Input: dimensioned drawing with shaded views. Units: mm. Origin: part minimum x, y, z. A direction names the side the tool comes from. Round coordinates to 2 decimals unless told otherwise and drop trailing zeros. Order: outer loops, then holes, each group sorted by start corner. A loop starts at its lowest first (then second) coordinate and runs counter-clockwise, first axis right, second up. Notation, with made-up numbers: M 11,-22.75 L 23,-22.75 A19 ccw 23,-12.75 Z; hole C 11,59 d1. An arc over 180 degrees is marked long. Put each result on its own line as item: value. Start each with the question number.
1) Section D-D, the plane y = 52.5. Return loops of the section in (x, z), then the cut area to 3 significant figures.
2) Access query for the marked faces 5 and 6. Directions: +Z, -Z, +X, -X, +Y, -Y. A direction counts if a zero-diameter tool reaches every point of the face in a straight line with its end or side. Return the directions, or none.
3) Section A-A, the plane z = 27.5. Return loops of the section in (x, y), then the cut area to 3 significant figures.
4) Section B-B, the plane y = 71. Return loops of the section in (x, z).
5) Draft query along X for the marked faces 1, 2, 3 and 4. Return one class per face: pulls with the +X half, pulls with the -X half, needs draft (parallel to the pull), parting line crosses it, or undercut.
6) Material intervals for probe 1 along Z at (x, y) = (26.15, 2.9); probe 2 along X at (y, z) = (2.05, 12.5); probe 3 along X at (y, z) = (7, 8), sorted ascending. Write a range as [from, to].
7) First-contact query: P1, Ø4, axis at x = 56.15, z = 42.5, coming from the +Y side. Flat tip, straight axial feed; report the tip coordinate or a pass-through.
8) Section C-C, the plane x = 56.15. Return loops of the section in (y, z).
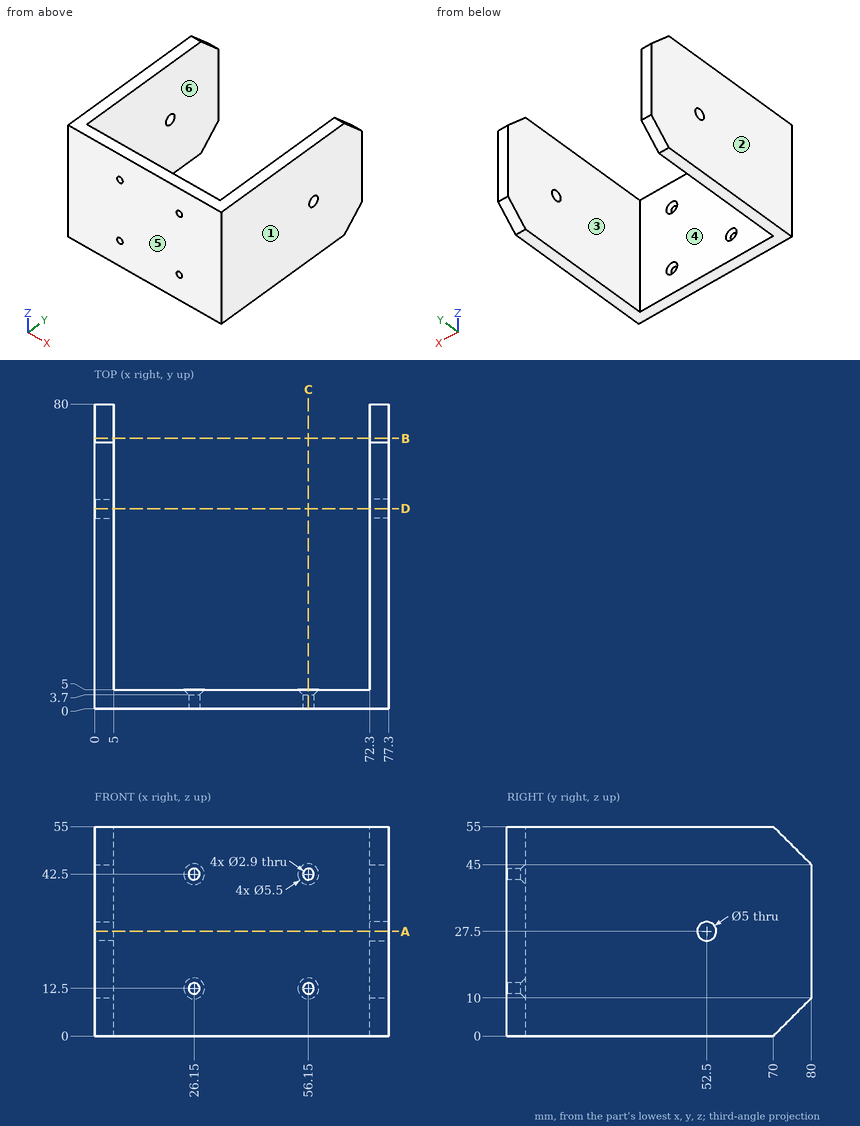
Result sheet:
1. outline: M 0,0 L 5,0 L 5,25 L 0,25 Z; M 0,30 L 5,30 L 5,55 L 0,55 Z; M 72.3,0 L 77.3,0 L 77.3,25 L 72.3,25 Z; M 72.3,30 L 77.3,30 L 77.3,55 L 72.3,55 Z
1. area: 500 mm2
2. face 5: +Z, -Z, +X, -X, -Y
2. face 6: +Z, -Z, +Y
3. outline: M 0,0 L 77.3,0 L 77.3,50 L 72.3,50 L 72.3,5 L 5,5 L 5,50 L 0,50 Z; M 0,55 L 5,55 L 5,80 L 0,80 Z; M 72.3,55 L 77.3,55 L 77.3,80 L 72.3,80 Z
3. area: 1,090 mm2
4. outline: M 0,1 L 5,1 L 5,54 L 0,54 Z; M 72.3,1 L 77.3,1 L 77.3,54 L 72.3,54 Z
5. face 1: pulls with the +X half
5. face 2: pulls with the -X half
5. face 3: undercut
5. face 4: undercut
6. probe 1: z = [0, 11.05], [13.95, 41.05], [43.95, 55]
6. probe 2: x = [0, 24.7], [27.6, 54.7], [57.6, 77.3]
6. probe 3: x = [0, 5], [72.3, 77.3]
7. P1: stops at y = 4.25
8. outline: M 0,0 L 5,0 L 5,9.75 L 3.7,11.05 L 0,11.05 Z; M 0,13.95 L 3.7,13.95 L 5,15.25 L 5,39.75 L 3.7,41.05 L 0,41.05 Z; M 0,43.95 L 3.7,43.95 L 5,45.25 L 5,55 L 0,55 Z
